Autodesk Inventor part; units mm, degrees
ref_plane "Work Plane1" through (-0.0014, -1.4859, 3.302) normal (-1, 0, 0) x (0, 0, 1)
ref_plane "YZ Plane" through (0, 0, 0) normal (1, 0, 0) x (0, 1, 0)
ref_plane "XZ Plane" through (0, 0, 0) normal (0, 1, 0) x (-1, 0, 0)
sketch "Sketch1" plane through (0, 0, 0) normal (0, 0, 1) x (1, 0, 0)
  line L0 (-3.9624, 3.8481) -> (3.9624, 3.8481)
  line L1 (3.9624, 3.8481) -> (3.9624, -3.8481)
  line L2 (3.9624, -3.8481) -> (-3.9624, -3.8481)
  line L3 (-3.9624, -3.8481) -> (-3.9624, 3.8481)
  line L4 (-3.9624, 3.8481) -> (3.9624, -3.8481) construction
  line L5 (3.9624, 3.8481) -> (-3.9624, -3.8481) construction
  point P0 (0, 0)
  dimension "d0" = 7.6962
  dimension "d1" = 7.9248
extrude "Extrusion1" add sketch "Sketch1" along normal blind 5.0038
sketch "Sketch4" plane through (-3.9624, 3.8481, 0) normal (0, 1, 0) x (1, 0, 0)
  line L0 (7.2277, -4.5029) -> (0.6971, -4.5029)
  line L1 (0.6971, -4.5029) -> (0.6971, -0.5009)
  line L2 (0.6971, -0.5009) -> (7.2277, -0.5009)
  line L3 (7.2277, -0.5009) -> (7.2277, -4.5029)
  line L4 (7.2277, -4.5029) -> (0.6971, -0.5009) construction
  line L5 (0.6971, -4.5029) -> (7.2277, -0.5009) construction
  line L6 (7.9248, -5.0038) -> (0, -5.0038)
  point P0 (3.9624, 0)
  point P1 (3.9624, -2.5019)
  dimension "d16" = 2.5019
extrude "Extrusion3" cut sketch "Sketch4" against normal blind 5.334
sketch "Sketch5" plane through (-3.9624, -3.8481, 0) normal (0, -1, 0) x (1, 0, 0)
  line L0 (7.9248, 5.0038) -> (0, 5.0038)
  line L1 (7.9248, 0) -> (0, 0)
  line L2 (0.6971, 5.0038) -> (7.2277, 5.0038)
  line L3 (7.2277, 5.0038) -> (7.2277, 0)
  line L4 (7.2277, 0) -> (0.6971, 0)
  line L5 (0.6971, 0) -> (0.6971, 5.0038)
  point P0 (3.9624, 0)
  point P1 (0.6971, 4.5029)
  point P2 (7.2277, 0.5009)
extrude "Extrusion4" cut sketch "Sketch5" against normal blind 1.905
sketch "Sketch9" plane through (0, 0, 5.0038) normal (0, 0, 1) x (1, 0, 0)
  line L0 (3.2653, 3.8481) -> (-3.2653, 3.8481)
  line L1 (-3.2653, -1.4859) -> (3.2653, -1.4859)
  line L2 (0.3773, 3.8481) -> (-0.3246, 3.8481)
  line L3 (-0.3246, 3.8481) -> (-0.3246, -1.4859)
  line L4 (-0.3246, -1.4859) -> (0.3773, -1.4859)
  line L5 (0.3773, -1.4859) -> (0.3773, 3.8481)
  line L6 (3.2653, 3.8481) -> (3.2653, -1.4859)
  line L7 (3.2653, -0.5528) -> (2.1497, -0.5528)
  line L8 (2.1497, -0.5528) -> (2.1497, 1.8689)
  line L9 (2.1497, 1.8689) -> (3.2653, 1.8689)
  line L10 (3.2653, 1.8689) -> (3.2653, -0.5528)
  line L11 (-3.2653, 3.8481) -> (-3.2653, -1.4859)
  line L12 (-3.2653, -0.5528) -> (-2.1497, -0.5528)
  line L13 (-2.1497, -0.5528) -> (-2.1497, 1.8689)
  line L14 (-2.1497, 1.8689) -> (-3.2653, 1.8689)
  line L15 (-3.2653, 1.8689) -> (-3.2653, -0.5528)
  point P0 (0, 0)
  dimension "d36" = 1.1156
  dimension "d37" = 1.1156
extrude "Extrusion7" cut sketch "Sketch9" against normal up to surface (0.5009 mm away) contours L5 L1 L3 L0 | L6 L7 L8 L9 | L14 L13 L12 L11
sketch "Sketch10" plane through (-3.9624, -1.4859, 0) normal (0, 1, 0) x (1, 0, 0)
  circle A0 centre (3.961, -3.302) radius 0.3937
  line L0 (7.9248, -5.0038) -> (4.3397, -5.0038)
  line L1 (0.6971, -4.5029) -> (0.6971, -0.5009)
  circle A1 centre (1.9544, -3.302) radius 0.3937
  line L2 (3.6378, -5.0038) -> (0, -5.0038)
  circle A2 centre (5.9676, -3.302) radius 0.3937
  point P0 (3.9624, 0)
  dimension "d40" = 1.7018
  dimension "d41" = 0.7874
  dimension "d42" = 3.2639
  dimension "d43" = 0.7874
  dimension "d44" = 1.7018
  dimension "d45" = 2.0066
  dimension "d46" = 0.7874
  dimension "d47" = 1.7018
  dimension "d48" = 2.0066
ref_plane "Work Plane1" through (-0.0014, -1.4859, 3.302) normal (-1, 0, 0) x (0, 0, 1)
sketch "Sketch11" plane through (-0.0014, -1.4859, 3.302) normal (-1, 0, 0) x (0, 0, 1)
  line L0 (-2.8011, 0) -> (1.2009, 0)
  line L1 (0.0001, 0) -> (0.0001, 4.334)
  line L2 (-2.8011, 5.334) -> (1.2009, 5.334)
  line L3 (-4.4984, -0.9144) -> (-6.604, -0.9144)
  line L4 (-3.302, -2.3622) -> (-3.302, 5.334)
  line L5 (-3.302, 5.334) -> (1.7018, 5.334)
  line L6 (-3.302, -0.9144) -> (-4.4984, -0.9144)
  line L7 (-3.302, -0.9144) -> (-0.5079, -0.9144)
  line L8 (0.0001, -0.4064) -> (0.0001, 0)
  arc A0 (-0.5079, -0.9144) -> (0.0001, -0.4064) centre (-0.5079, -0.4064) ccw
  point P0 (-3.302, 1.4859)
  dimension "d49" = 1
  dimension "d50" = 3.302
  dimension "d51" = 6.2484
  dimension "d52" = 0.508
sweep "Sweep1" add profiles "Sketch10" path "Sketch11" path curves L3 L6 L7 A0 L8 L1
sketch "Sketch12" plane through (3.9624, -3.8481, 0) normal (1, 0, 0) x (0, 0, -1)
  line L0 (-4.5029, 7.6962) -> (-0.5009, 7.6962)
  line L1 (-3.8364, 7.6962) -> (-2.7933, 7.6962)
  line L2 (-2.7933, 7.6962) -> (-2.7933, 5.3015)
  line L3 (-2.7933, 5.3015) -> (-3.8364, 5.3015)
  line L4 (-3.8364, 5.3015) -> (-3.8364, 7.6962)
  point P0 (0, 3.8481)
extrude "Extrusion8" cut sketch "Sketch12" against normal up to surface (0.6971 mm away)
sketch "Sketch13" plane through (-3.9624, -3.8481, 0) normal (-1, 0, 0) x (0, 0, 1)
  line L0 (3.8364, 7.6962) -> (4.5029, 7.6962)
  line L1 (2.7933, 5.3015) -> (2.7933, 7.6962)
  line L2 (3.8364, 7.6962) -> (2.7933, 7.6962)
  line L3 (2.7933, 7.6962) -> (2.7933, 5.3015)
  line L4 (2.7933, 5.3015) -> (3.8364, 5.3015)
  line L5 (3.8364, 5.3015) -> (3.8364, 7.6962)
  point P0 (0, 3.8481)
extrude "Extrusion9" cut sketch "Sketch13" against normal up to surface (0.6971 mm away)
equation "\"d37\" = d36"
equation "\"d44\" = d40"
equation "\"d47\" = d40"
equation "\"d48\" = d45"
properties part number "2SH-C-03-TR"
Geometry check sheet. Reference: the model listing, model coordinates, mm. A direction names the side the tool comes from. Round coordinates to 2 decimals unless told otherwise and drop trailing zeros. Write each loop counter-clockwise with the first axis right and the second up, starting at its lowest first coordinate (ties: lowest second). Pieces come first, ordered by that corner, then holes. Notation, with made-up numbers: (-28, 34.5) -> (0, 34.5) arc R30 cw to (0, 65.5) -> close; hole circle Ø2 at (32.5, 36.5). An arc over 180 degrees is marked (long way). Put each result on its own line as item: value.
1) Cross-section at C-C, the plane y = 0.75. Enter the section's corners in (x, z), plus the area to 3 significant figures.
Recorded:
outline: (-3.96, 0) -> (3.96, 0) -> (3.96, 5) -> (3.27, 5) -> (3.27, 0.5) -> (-3.27, 0.5) -> (-3.27, 5) -> (-3.96, 5) -> close; circle Ø0.79 at (-2.01, 3.3); (-2.15, 4.5) -> (-0.32, 4.5) -> (-0.32, 5) -> (-2.15, 5) -> close; circle Ø0.79 at (0, 3.3); (0.38, 4.5) -> (2.15, 4.5) -> (2.15, 5) -> (0.38, 5) -> close; circle Ø0.79 at (2.01, 3.3)
area: 13.5 mm2
2) Cross-section at A-A, the plane y = -3. Enter the section's corners in (x, z).
Recorded:
outline: (-3.96, 0) -> (-3.27, 0) -> (-3.27, 5) -> (-3.96, 5) -> close; (3.27, 0) -> (3.96, 0) -> (3.96, 5) -> (3.27, 5) -> close
3) Release check for a two-part mould opening along Z. For faces 1 (the face through (0, 1, 0)), 2 (the face through (1.5, 1.2, 4.503)), 3 (the face through (-3.962, 0, 2)) record: pulls with the +Z half, pulls with the -Z half, needs draft (parallel to the pull), parting line crosses it, or undercut.
Recorded:
face 1: pulls with the -Z half
face 2: undercut
face 3: needs draft
4) Cross-section at D-D, the plane y = 3. Enter the section's corners in (x, z), plus the area to 3 significant figures.
Recorded:
outline: (-3.96, 0) -> (3.96, 0) -> (3.96, 2.79) -> (3.27, 2.79) -> (3.27, 0.5) -> (-3.27, 0.5) -> (-3.27, 2.79) -> (-3.96, 2.79) -> close; (-3.96, 3.84) -> (-3.27, 3.84) -> (-3.27, 4.5) -> (-0.32, 4.5) -> (-0.32, 5) -> (-3.96, 5) -> close; (0.38, 4.5) -> (3.27, 4.5) -> (3.27, 3.84) -> (3.96, 3.84) -> (3.96, 5) -> (0.38, 5) -> close
area: 11.7 mm2
5) Access from +Z, -Z, +X, -X, +Y, -Y to the whole of each face (thin tool, end or side, straight path). Record for faces 4 (the face through (3.962, 0, 2)), 5 (the face through (-3.265, -3, 2)), 6 (the face through (-1, 1, 4.503)).
Recorded:
face 4: +Z, -Z, +X, +Y, -Y
face 5: +Z, -Z, -Y
face 6: +Y
6) Depth check by flat-ended pin: P1, Ø0.6, axis at x = 0, z = 3.5, coming from the +Y side; P2, Ø0.6, axis at x = -2.5, z = 5, coming from the -Y side; P3, Ø0.9, axis at x = -1, y = 1, coming from the -Z side. Enter the tip coordinate at first touch or a pass-through.
Recorded:
P1: stops at y = 2.85
P2: stops at y = -1.94
P3: stops at z = 0
7) Cross-section at B-B, the plane x = 3. Enter the section's corners in (y, z), plus the area to 3 significant figures.
Recorded:
outline: (-1.94, 0) -> (3.85, 0) -> (3.85, 0.5) -> (-1.49, 0.5) -> (-1.49, 4.5) -> (-0.55, 4.5) -> (-0.55, 5) -> (-1.94, 5) -> close; (1.87, 4.5) -> (3.85, 4.5) -> (3.85, 5) -> (1.87, 5) -> close
area: 6.42 mm2
8) Thickness scan on probe 1 along X at (y, z) = (-0.25, 2.75); probe 2 along Z at (x, y) = (2.5, 3); probe 3 along X at (y, z) = (-2, 3). Record the ranges inside material, lowest first. Write a range as from..to.
Recorded:
probe 1: x = -3.96..-3.27, 3.27..3.96
probe 2: z = 0..0.5, 4.5..5
probe 3: x = -3.96..-3.27, -2.29..-1.73, -0.28..0.28, 1.72..2.29, 3.27..3.96
